Geometry: final body of the model. Coordinates: model frame, mm. Face numbers are marked on the shaded views. A direction names the side the tool comes from. Give positions to 0.01 mm unless a question says otherwise; leave off trailing zeros. Write each loop counter-clockwise with the first axis right and the second up, starting at its lowest first coordinate (ties: lowest second). Pieces come first, ordered by that corner, then holes. Notation, with made-up numbers: (61, 66.25) - (68, 66.25) arc R25 ccw to (68, 104.25) - close; hole circle Ø1 at (-20, 21). An arc over 180 degrees is marked (long way). Return JSON: item names as keys, results as strings.
from build123d import *

# Parameters (mm, degrees)
F0_W     = 172.72
F0_H     = 66.548
F1_DEPTH = 63.5
F2_W     = 150.368
F2_H     = 22.352
F3_DEPTH = 189.62974
F4_W     = 150.368
F4_H     = 66.548
F5_DEPTH = 22.53701
F6_DEPTH = 63.5
F7_DEPTH = 41.45952
F8_DEPTH = 3.37497


with BuildPart() as f1:
    # F0 (on Top) → F1 (new body)
    with BuildSketch(Plane.XY):
        Rectangle(F0_W, F0_H)
    extrude(amount=F1_DEPTH)

    # F2 (on face) → F3 (cut)
    with BuildSketch(Plane.XZ.offset(33.274)):
        with Locations((-11.176, 11.176)):
            Rectangle(F2_W, F2_H)
    extrude(amount=-F3_DEPTH, mode=Mode.SUBTRACT)

    # F4 (on face) → F5 (cut)
    with BuildSketch(Plane.XY.offset(63.5)):
        with Locations((11.176, 0)):
            Rectangle(F4_W, F4_H)
    extrude(amount=-F5_DEPTH, mode=Mode.SUBTRACT)

    # F6 (add): a face of the model
    f6_faces = [f1.faces().sort_by_distance(p)[0] for p in [
        (-75.184, 0, 63.5),
    ]]
    extrude(f6_faces, amount=F6_DEPTH)

    # F7 (cut): a face of the model
    f7_faces = [f1.faces().sort_by_distance(p)[0] for p in [
        (-75.184, 0, 127),
    ]]
    extrude(f7_faces, amount=-F7_DEPTH, mode=Mode.SUBTRACT)

    # F8 (cut): a face of the model
    f8_faces = [f1.faces().sort_by_distance(p)[0] for p in [
        (-75.184, 0, 85.54048),
    ]]
    extrude(f8_faces, amount=-F8_DEPTH, mode=Mode.SUBTRACT)


solid = f1.part
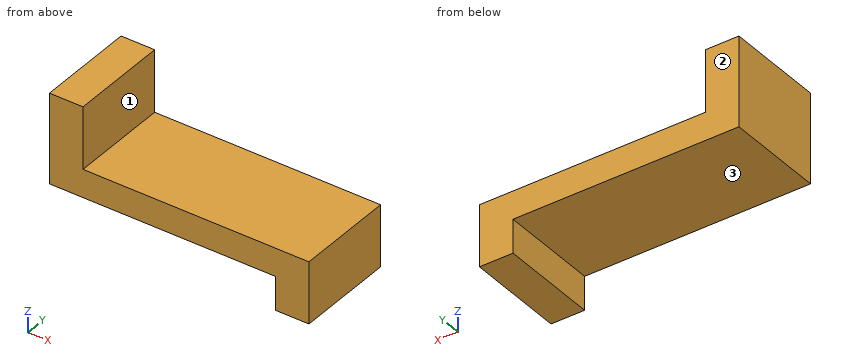
Q1. Set-up query: the marked faces 1, 2 and 3. Return all of +Z, -Z, +X, -X, +Y, -Y with unobstructed straight access to the full face (end or side cutting, diameter ignored); none if empty.
Answer key:
{"face 1": "+Z, +X, +Y, -Y", "face 2": "+Z, -Z, +X, -X, +Y", "face 3": "-Z, -X, +Y, -Y"}
Q2. Section query C-C, the plane z = 11. Return the cut outline in (x, y), plus the area to 3 significant figures.
Answer key:
{"outline": "(64.01, -33.27) - (86.36, -33.27) - (86.36, 33.27) - (64.01, 33.27) - close", "area": "1,490 mm^2"}
Q3. Section query A-A, the plane y = -27. Return the cut outline in (x, z), plus the area to 3 significant figures.
Answer key:
{"outline": "(-86.36, 22.35) - (64.01, 22.35) - (64.01, 0) - (86.36, 0) - (86.36, 40.96) - (-64.01, 40.96) - (-64.01, 82.17) - (-86.36, 82.17) - close", "area": "4,640 mm^2"}
Q4. Pin query (flat end, axial travel): P1, Ø1.5, axis at y = -11.5, z = 14, coming from the -X side; P2, Ø20.5, axis at y = -14, z = 56.5, coming from the +X side; P3, Ø10, axis at x = -50, y = -22, coming from the +Z side. Return the tip coordinate at first contact, or that it passes through.
Answer key:
{"P1": "stops at x = 64.01", "P2": "stops at x = -64.01", "P3": "stops at z = 40.96"}
Q5. Material intervals for probe 1 along Z at (x, y) = (-59.5, 0.5); probe 2 along X at (y, z) = (18, 56); probe 3 along Z at (x, y) = (-68, -22.5), sorted ascending. Write a range as [from, to].
Answer key:
{"probe 1": "z = [22.35, 40.96]", "probe 2": "x = [-86.36, -64.01]", "probe 3": "z = [22.35, 82.17]"}
Q6. Section query B-B, the plane x = -74. Return the cut outline in (y, z), plus the area to 3 significant figures.
Answer key:
{"outline": "(-33.27, 22.35) - (33.27, 22.35) - (33.27, 82.17) - (-33.27, 82.17) - close", "area": "3,980 mm^2"}
